from build123d import *

# Parameters (mm, degrees)
EXTRUDE_1_DEPTH     = 10
SKETCH_2_R          = 1.6
CUT_EXTRUDE_1_DEPTH = 10
EXTRUDE_2_DEPTH     = 10


with BuildPart() as part:
    # 草图1 → 凸台-拉伸1 (new body)
    with BuildSketch(Plane.XY):
        with BuildLine():
            ThreePointArc((-14.346020253, 3.273810573), (-12.969870434, 2.10791515), (-11.273952779, 1.493941396))
            ThreePointArc((-11.273952779, 1.493941396), (-11.372074296, 0.730383496), (-11.41592688, -0.03820316))
            ThreePointArc((-11.41592688, -0.03820316), (-13.195785695, -0.330098793), (-14.762736671, -1.223275765))
            ThreePointArc((-14.762736671, -1.223275765), (-14.733672875, -1.587766767), (-14.695266759, -1.951392075))
            ThreePointArc((-14.695266759, -1.951392075), (-12.990875263, -2.541434526), (-11.187686245, -2.501311882))
            ThreePointArc((-11.187686245, -2.501311882), (-11.003352906, -3.248753999), (-10.766598699, -3.981281092))
            ThreePointArc((-10.766598699, -3.981281092), (-12.320822752, -4.896424828), (-13.459308284, -6.295335531))
            ThreePointArc((-13.459308284, -6.295335531), (-13.300537764, -6.624714214), (-13.133368515, -6.949910827))
            ThreePointArc((-13.133368515, -6.949910827), (-11.33092286, -6.884411803), (-9.663993147, -6.195611546))
            ThreePointArc((-9.663993147, -6.195611546), (-9.222100192, -6.825991681), (-8.736714161, -7.423527369))
            ThreePointArc((-8.736714161, -7.423527369), (-9.855396881, -8.838323974), (-10.411658189, -10.554037767))
            ThreePointArc((-10.411658189, -10.554037767), (-10.144623785, -10.803819715), (-9.871268536, -11.046668027))
            ThreePointArc((-9.871268536, -11.046668027), (-8.214198994, -10.334473534), (-6.908656681, -9.090021956))
            ThreePointArc((-6.908656681, -9.090021956), (-6.268884202, -9.518203778), (-5.600420419, -9.900047555))
            ThreePointArc((-5.600420419, -9.900047555), (-6.132477506, -11.62342091), (-6.031388419, -13.424221137))
            ThreePointArc((-6.031388419, -13.424221137), (-5.692154606, -13.560671914), (-5.349531499, -13.688373915))
            ThreePointArc((-5.349531499, -13.688373915), (-4.061634494, -12.425669766), (-3.293800304, -10.793636948))
            ThreePointArc((-3.293800304, -10.793636948), (-2.542553119, -10.96179213), (-1.781291324, -11.076373878))
            ThreePointArc((-1.781291324, -11.076373878), (-1.65486552, -12.87557286), (-0.910078679, -14.518251473))
            ThreePointArc((-0.910078679, -14.518251473), (-0.544460863, -14.522942645), (-0.178843046, -14.518251473))
            ThreePointArc((-0.178843046, -14.518251473), (0.565943794, -12.87557286), (0.692369599, -11.076373878))
            ThreePointArc((0.692369599, -11.076373878), (1.453631394, -10.96179213), (2.204878579, -10.793636948))
            ThreePointArc((2.204878579, -10.793636948), (2.972712769, -12.425669766), (4.260609774, -13.688373915))
            ThreePointArc((4.260609774, -13.688373915), (4.603232881, -13.560671914), (4.942466694, -13.424221137))
            ThreePointArc((4.942466694, -13.424221137), (5.043555781, -11.62342091), (4.511498694, -9.900047555))
            ThreePointArc((4.511498694, -9.900047555), (5.179962477, -9.518203778), (5.819734956, -9.090021956))
            ThreePointArc((5.819734956, -9.090021956), (7.125277269, -10.334473534), (8.782346811, -11.046668027))
            ThreePointArc((8.782346811, -11.046668027), (9.055702059, -10.803819715), (9.322736464, -10.554037767))
            ThreePointArc((9.322736464, -10.554037767), (8.766475155, -8.838323974), (7.647792436, -7.423527369))
            ThreePointArc((7.647792436, -7.423527369), (8.133178467, -6.825991681), (8.575071422, -6.195611546))
            ThreePointArc((8.575071422, -6.195611546), (10.242001135, -6.884411803), (12.04444679, -6.949910827))
            ThreePointArc((12.04444679, -6.949910827), (12.211616039, -6.624714214), (12.370386559, -6.295335531))
            ThreePointArc((12.370386559, -6.295335531), (11.231901027, -4.896424828), (9.677676974, -3.981281092))
            ThreePointArc((9.677676974, -3.981281092), (9.914431181, -3.248753999), (10.09876452, -2.501311882))
            ThreePointArc((10.09876452, -2.501311882), (11.901953538, -2.541434526), (13.606345034, -1.951392075))
            ThreePointArc((13.606345034, -1.951392075), (13.64475115, -1.587766767), (13.673814946, -1.223275765))
            ThreePointArc((13.673814946, -1.223275765), (12.10686397, -0.330098793), (10.327005155, -0.03820316))
            ThreePointArc((10.327005155, -0.03820316), (10.28315257, 0.730383496), (10.185031054, 1.493941396))
            ThreePointArc((10.185031054, 1.493941396), (11.880948709, 2.10791515), (13.257098528, 3.273810573))
            ThreePointArc((13.257098528, 3.273810573), (13.161554553, 3.626754964), (13.056986399, 3.977131755))
            ThreePointArc((13.056986399, 3.977131755), (11.273195392, 4.243946496), (9.50808161, 3.873171904))
            ThreePointArc((9.50808161, 3.873171904), (9.189544768, 4.574016236), (8.822220251, 5.250567193))
            ThreePointArc((8.822220251, 5.250567193), (10.181823465, 6.435716787), (11.04387495, 8.020004545))
            ThreePointArc((11.04387495, 8.020004545), (10.827284626, 8.314600924), (10.603207031, 8.603543177))
            ThreePointArc((10.603207031, 8.603543177), (8.843486852, 8.207960878), (7.3315065, 7.224591224))
            ThreePointArc((7.3315065, 7.224591224), (6.781305566, 7.763040321), (6.19438726, 8.26121238))
            ThreePointArc((6.19438726, 8.26121238), (7.034054087, 9.857476795), (7.265582407, 11.646190047))
            ThreePointArc((7.265582407, 11.646190047), (6.957197458, 11.84265154), (6.643873342, 12.031136003))
            ThreePointArc((6.643873342, 12.031136003), (5.145883953, 11.026582245), (4.091238356, 9.563427049))
            ThreePointArc((4.091238356, 9.563427049), (3.383681016, 9.866760378), (2.65643549, 10.119272641))
            ThreePointArc((2.65643549, 10.119272641), (2.86276427, 11.911067522), (2.432500244, 13.662630633))
            ThreePointArc((2.432500244, 13.662630633), (2.073969766, 13.734424026), (1.713715288, 13.796994828))
            ThreePointArc((1.713715288, 13.796994828), (0.679768455, 12.319140163), (0.224893345, 10.573806643))
            ThreePointArc((0.224893345, 10.573806643), (-0.544460863, 10.601057355), (-1.31381507, 10.573806643))
            ThreePointArc((-1.31381507, 10.573806643), (-1.76869018, 12.319140163), (-2.802637013, 13.796994828))
            ThreePointArc((-2.802637013, 13.796994828), (-3.162891491, 13.734424026), (-3.521421969, 13.662630633))
            ThreePointArc((-3.521421969, 13.662630633), (-3.951685995, 11.911067522), (-3.745357215, 10.119272641))
            ThreePointArc((-3.745357215, 10.119272641), (-4.472602741, 9.866760378), (-5.180160081, 9.563427049))
            ThreePointArc((-5.180160081, 9.563427049), (-6.234805678, 11.026582245), (-7.732795067, 12.031136003))
            ThreePointArc((-7.732795067, 12.031136003), (-8.046119184, 11.84265154), (-8.354504132, 11.646190047))
            ThreePointArc((-8.354504132, 11.646190047), (-8.122975812, 9.857476795), (-7.283308985, 8.26121238))
            ThreePointArc((-7.283308985, 8.26121238), (-7.870227292, 7.763040321), (-8.420428225, 7.224591224))
            ThreePointArc((-8.420428225, 7.224591224), (-9.932408577, 8.207960878), (-11.692128756, 8.603543177))
            ThreePointArc((-11.692128756, 8.603543177), (-11.916206351, 8.314600924), (-12.132796675, 8.020004545))
            ThreePointArc((-12.132796675, 8.020004545), (-11.27074519, 6.435716787), (-9.911141976, 5.250567193))
            ThreePointArc((-9.911141976, 5.250567193), (-10.278466493, 4.574016236), (-10.597003335, 3.873171904))
            ThreePointArc((-10.597003335, 3.873171904), (-12.362117117, 4.243946496), (-14.145908124, 3.977131755))
            ThreePointArc((-14.145908124, 3.977131755), (-14.250476278, 3.626754964), (-14.346020253, 3.273810573))
        make_face()
    extrude(amount=EXTRUDE_1_DEPTH)

    # 草图2 → 切除-拉伸1 (cut)
    with BuildSketch(Plane.XY.offset(10)):
        Circle(SKETCH_2_R)
    extrude(amount=-CUT_EXTRUDE_1_DEPTH, mode=Mode.SUBTRACT)

    # 草图3 → 凸台-拉伸2 (add)
    with BuildSketch(Plane.XY.offset(10)):
        with BuildLine():
            Line((-35.145602395, -19.299750751), (-6.268884202, -9.518203778))
            Line((-6.268884202, -9.518203778), (-11.187686245, -2.501311882))
            Line((-11.187686245, -2.501311882), (-31.902692825, -9.518203778))
            ThreePointArc((-31.902692825, -9.518203778), (-55.564328736, -9.890192083), (-71.354077075, 7.736357117))
            Line((-71.354077075, 7.736357117), (-71.354077075, 0))
            Line((-71.354077075, 0), (-68.451868042, -8.25925779))
            Line((-68.451868042, -8.25925779), (-66.492126744, -13.648546361))
            Line((-66.492126744, -13.648546361), (-35.145602395, -19.299750751))
        make_face()
    extrude(amount=-EXTRUDE_2_DEPTH)


solid = part.part
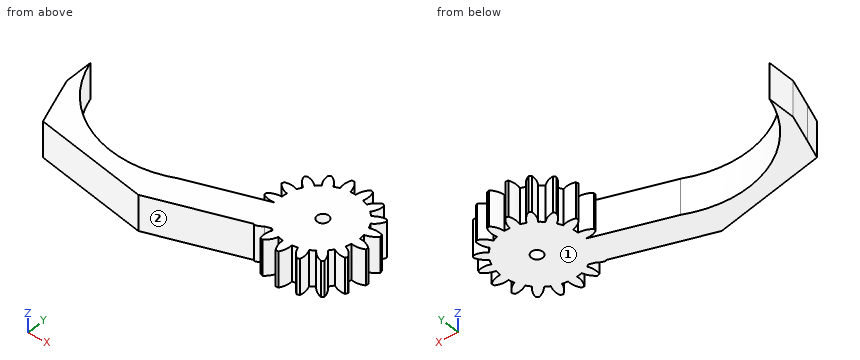
Verification items for the finished model (mm, model axes). Face numbers are marked on the shaded views. A direction names the side the tool comes from. Coordinates: 2 decimals unless noted, no trailing zeros. Order: outer loops, then holes, each group sorted by start corner. A loop starts at its lowest first (then second) coordinate and runs counter-clockwise, first axis right, second up. Notation, with made-up numbers: M -13.75,52.25 L 30.25,52.25 A25 ccw 30.25,89.25 Z; hole C 36.25,16.5 d9. An arc over 180 degrees is marked long. One line per item, written item: value. Start each with the question number.
Item 1: Sectioned sample at C-C (x = -43.5). Enter the section's corners in (y, z), then the cut area to 3 significant figures.
Item 2: Access from +Z, -Z, +X, -X, +Y, -Y to the whole of each face (thin tool, end or side, straight path). Record for the marked faces 1 and 2.
Item 3: Sectioned sample at A-A (y = -5). Enter the section's corners in (x, z).
Item 4: Gauge pin test, flat ends, axial feed: pin 1 (1.5 mm diameter, centred on y = 10.5, z = 5.5, fed in from +X); pin 2 (5 mm diameter, centred on y = -6, z = 3, fed in from -X); pin 3 (2 mm diameter, centred on y = 0, z = 6, fed in from +X). Record the tip position at first contact, or that the pin passes through.
Item 5: Scan lines: probe 1 along X at (y, z) = (0.5, 1.5); probe 2 along Y at (x, z) = (-14, 9.25); probe 3 along X at (y, z) = (2.5, 6) (3 decimals). Record each from-to range of solid material in increasing order.
Item 6: Sectioned sample at B-B (x = -23). Enter the section's corners in (y, z), then the cut area to 3 significant figures.
Conclusion:
1. outline: M -17.79,0 L -12.27,0 L -12.27,10 L -17.79,10 Z
1. area: 55.2 mm^2
2. face 1: -Z, +X, -X, +Y, -Y
2. face 2: +Z, -Z, -Y
3. outline: M -69.6,0 L -63.17,0 L -63.17,10 L -69.6,10 Z; M -18.56,0 L 11.35,0 L 11.35,10 L -18.56,10 Z
4. pin 1: stops at x = 7.27
4. pin 2: stops at x = -70.12
4. pin 3: stops at x = 13.39
5. probe 1: x = -71.35 to -67.92, -11.39 to -1.52, 1.52 to 10.3
5. probe 2: y = -12.14 to -3.45, -2.28 to -0.7, 2.9 to 4.02
5. probe 3: x = -71.354 to -69.125, -13.551 to 12.462
6. outline: M -15.19,0 L -6.5,0 L -6.5,10 L -15.19,10 Z
6. area: 86.8 mm^2
